Design review of the part shown in the three views and the two pictorial views. Dimensions are in mm from the part's minimum x, y and z. A direction names the side the tool comes from. Coordinates: 2 decimals unless noted, no trailing zeros. Write each loop counter-clockwise with the first axis right and the second up, starting at its lowest first coordinate (ties: lowest second). Pieces come first, ordered by that corner, then holes.
Q1. For L1, parallel to Y at x = 16.5, z = 1.65; L2, parallel to X at y = 7.25, z = 0.25, list the stretches that pass through material, from the lowest coordinate up.
Q2. Take a section at B-B, the plane x = 26. Write out the cut boundary in (y, z).
Q3. For pin 1 Ø1.5 at (x, z) = (27.5, 1.5) entering from -Y; pin 2 Ø0.9 at (y, z) = (5.5, 1.5) entering from -X, all flat-tipped, find the tip position at first contact; note any pin that passes through.
Q4. For the marked faces 1 and 2, list the 3-axis set-ups (+Z, -Z, +X, -X, +Y, -Y) from which the entire face can be reached by the end or side of a thin tool; tool diameter is ignored.
Q5. Take a section at C-C, the plane z = 0.7. State how many separate pieces and enclosed holes the cut face has, plus the area to 4 significant figures.
Q6. Take a section at A-A, the plane y = 15. Write out the cut boundary in (x, z), plus the area to 3 significant figures.
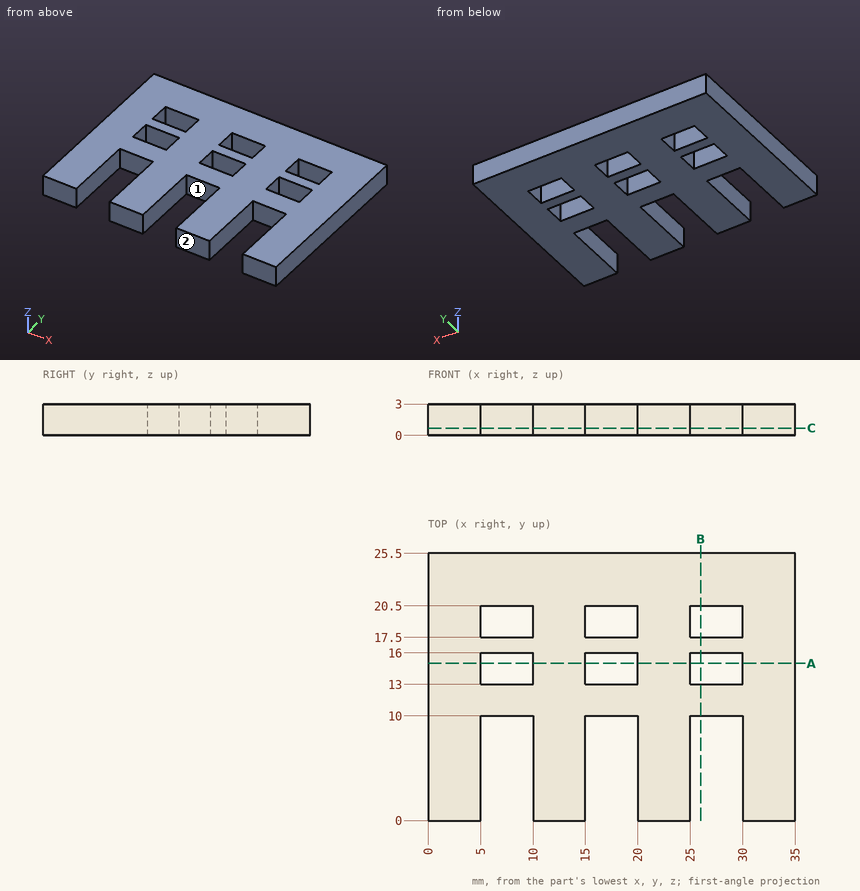
Responses:
1. L1: y = 10 to 13, 16 to 17.5, 20.5 to 25.5
1. L2: x = 0 to 5, 10 to 15, 20 to 25, 30 to 35
2. outline: (10, 0) - (13, 0) - (13, 3) - (10, 3) - close; (16, 0) - (17.5, 0) - (17.5, 3) - (16, 3) - close; (20.5, 0) - (25.5, 0) - (25.5, 3) - (20.5, 3) - close
3. pin 1: stops at y = 10
3. pin 2: stops at x = 0
4. face 1: +Z, -Z, -Y
4. face 2: +Z, -Z, +X, -X, -Y
5. separate pieces: 1
5. enclosed holes: 6
5. area: 652.5 mm2
6. outline: (0, 0) - (5, 0) - (5, 3) - (0, 3) - close; (10, 0) - (15, 0) - (15, 3) - (10, 3) - close; (20, 0) - (25, 0) - (25, 3) - (20, 3) - close; (30, 0) - (35, 0) - (35, 3) - (30, 3) - close
6. area: 60.0 mm2
